The model under review builds one solid part; all positions refer to its coordinate system, in mm. Round coordinates to 2 decimals unless told otherwise and drop trailing zeros.
1) Consider section A-A (z = 2.75). Give the number of separate pieces and of enclosed holes in the cut face, then the cut area to 3 significant figures.
2) To check wall thickness, follow L1, parallel to X at y = 6, z = 4; L2, parallel to Y at x = 56, z = 5.5; L3, parallel to Y at x = -28.5, z = 2.25. State the ranges of each line that lie inside material, in increasing order.
3) Clearance check with a flat-ended pin moving along its axis: P1, Ø5.5, axis at x = 56.388, y = 13.081, coming from the +Z side. State where the tip first meets the part, or that it passes through.
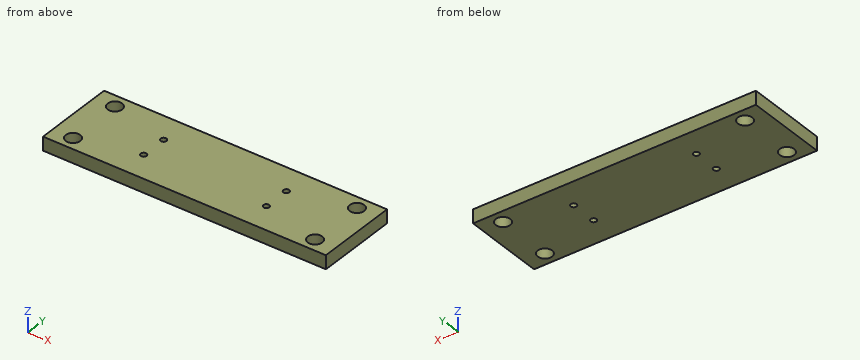
from build123d import *

# Parameters (mm, degrees)
SKETCH1_W               = 131.826
SKETCH1_H               = 38.1
BOSS_EXTRUDE1_DEPTH     = 6.35
F_1_4_CLEARANCE_HOLE1_D = 6.7564
F_6_32_TAPPED_HOLE1_D   = 2.7051


with BuildPart() as part:
    # Sketch1 → Boss-Extrude1 (new body)
    with BuildSketch(Plane.XY):
        Rectangle(SKETCH1_W, SKETCH1_H)
    extrude(amount=BOSS_EXTRUDE1_DEPTH)

    # 1/4 Clearance Hole1 (through all)
    with Locations(Plane.XY.offset(6.35)):
        with Locations((-56.388, 13.081), (-56.388, -13.081)):
            f_1_4_clearance_hole1 = Hole(F_1_4_CLEARANCE_HOLE1_D / 2)

    # #6-32 Tapped Hole1 (through all)
    with Locations(Plane.XY.offset(6.35)):
        with Locations((-28.575, 6.2103), (-28.575, -6.2103)):
            f_6_32_tapped_hole1 = Hole(F_6_32_TAPPED_HOLE1_D / 2)

    # Mirror1: 1/4 Clearance Hole1, #6-32 Tapped Hole1 across plane
    add(f_1_4_clearance_hole1.mirror(Plane(origin=(0, 0, 0), x_dir=(0, 0, 1), z_dir=(1, 0, 0))), mode=Mode.SUBTRACT)
    add(f_6_32_tapped_hole1.mirror(Plane(origin=(0, 0, 0), x_dir=(0, 0, 1), z_dir=(1, 0, 0))), mode=Mode.SUBTRACT)


solid = part.part
Answer below:
1. separate pieces: 1
1. enclosed holes: 8
1. area: 4,860 mm2
2. L1: x = -65.91 to -29.91, -27.24 to 27.24, 29.91 to 65.91
2. L2: y = -19.05 to -16.44, -9.73 to 9.73, 16.44 to 19.05
2. L3: y = -19.05 to -7.56, -4.86 to 4.86, 7.56 to 19.05
3. P1: passes through
